Geometry check sheet. Reference: the model listing, model coordinates, mm. A direction names the side the tool comes from. Round coordinates to 2 decimals unless told otherwise and drop trailing zeros. Order: outer loops, then holes, each group sorted by start corner. A loop starts at its lowest first (then second) coordinate and runs counter-clockwise, first axis right, second up. Notation, with made-up numbers: M 32,45.25 L 68,45.25 A15 ccw 68,49.25 Z; hole C 56.25,-14.75 d9. An arc over 180 degrees is marked long. Return JSON: item names as keys, results as strings. Group by question number.
```python
from build123d import *

# Parameters (mm, degrees)
SKETCH1_W           = 70
SKETCH1_H           = 31.9
BOSS_EXTRUDE1_DEPTH = 3
SKETCH2_R           = 1.2
CUT_EXTRUDE1_DEPTH  = 3
SKETCH3_W           = 24
SKETCH3_H           = 22.6
CUT_EXTRUDE2_DEPTH  = 3


with BuildPart() as part:
    # Sketch1 → Boss-Extrude1 (new body)
    with BuildSketch(Plane(origin=(0, 0, 0), x_dir=(1, 0, 0), z_dir=(0, 1, 0))):
        Rectangle(SKETCH1_W, SKETCH1_H)
    extrude(amount=BOSS_EXTRUDE1_DEPTH)

    # Sketch2 → Cut-Extrude1 (cut)
    with BuildSketch(Plane(origin=(0, 3, 0), x_dir=(1, 0, 0), z_dir=(0, 1, 0))):
        with Locations((-29, 13.65)):
            Circle(SKETCH2_R)
    cut_extrude1 = extrude(amount=-CUT_EXTRUDE1_DEPTH, mode=Mode.SUBTRACT)

    # Mirror1: Cut-Extrude1 across plane
    add(cut_extrude1.mirror(Plane.XY), mode=Mode.SUBTRACT)

    # Sketch3 → Cut-Extrude2 (cut)
    with BuildSketch(Plane(origin=(0, 3, 0), x_dir=(1, 0, 0), z_dir=(0, 1, 0))):
        with Locations((-35, 0)):
            Rectangle(SKETCH3_W, SKETCH3_H)
    extrude(amount=-CUT_EXTRUDE2_DEPTH, mode=Mode.SUBTRACT)


solid = part.part
```
Q1. Depth check by flat-ended pin: pin 1 Ø4 at (x, z) = (-1, -0.5) entering from -Y. Enter the tip coordinate at first touch or a pass-through.
Q2. Section check B-B on y = 1.2. Record the cut outline in (x, z), plus the area to 3 significant figures.
Q3. Set-up check for faces 4 (the face through (7, 0, 0)), 5 (the face through (-23, 2, 0)): record each of +Z, -Z, +X, -X, +Y, -Y from which the full face is reachable in a straight line by a thin tool's end or side.
Q4. Release check for a two-part mould opening along Z. For faces 1 (the face through (-28.35, 1.52, 14.66)), 2 (the face through (35, 1, 0)), 3 (the face through (0, 1, 15.95)) record: +Z half, -Z half, draft (parallel to the pull), parting line (faces both ways), or undercut.
Q5. Section check C-C on z = 13.65. Record the cut outline in (x, y), plus the area to 3 significant figures.
Q6. Section check D-D on z = 0. Record the cut outline in (x, y), plus the area to 3 significant figures.
Q7. Section check A-A on x = -29. Record the cut outline in (y, z), plus the area to 3 significant figures.
Q8. Material ranges on line 1 along Z through (x, y) = (-29, 1.45); line 2 along X through (y, z) = (1.55, -13.65); line 3 along X through (y, z) = (2.3, -6), recorded low to high.
Geometry check:
{
 "1": {"pin 1": "stops at y = 0"},
 "2": {"outline": "M -35,-15.95 L 35,-15.95 L 35,15.95 L -35,15.95 L -35,11.3 L -23,11.3 L -23,-11.3 L -35,-11.3 Z; hole C -29,-13.65 d2.4; hole C -29,13.65 d2.4", "area": "1,950 mm^2"},
 "3": {"face 4": "+Z, -Z, +X, -X, -Y", "face 5": "-X, +Y, -Y"},
 "4": {"face 1": "undercut", "face 2": "draft", "face 3": "+Z half"},
 "5": {"outline": "M -35,0 L -30.2,0 L -30.2,3 L -35,3 Z; M -27.8,0 L 35,0 L 35,3 L -27.8,3 Z", "area": "203 mm^2"},
 "6": {"outline": "M -23,0 L 35,0 L 35,3 L -23,3 Z", "area": "174 mm^2"},
 "7": {"outline": "M 0,-15.95 L 3,-15.95 L 3,-14.85 L 0,-14.85 Z; M 0,-12.45 L 3,-12.45 L 3,-11.3 L 0,-11.3 Z; M 0,11.3 L 3,11.3 L 3,12.45 L 0,12.45 Z; M 0,14.85 L 3,14.85 L 3,15.95 L 0,15.95 Z", "area": "13.5 mm^2"},
 "8": {"line 1": "z = -15.95 to -14.85, -12.45 to -11.3, 11.3 to 12.45, 14.85 to 15.95", "line 2": "x = -35 to -30.2, -27.8 to 35", "line 3": "x = -23 to 35"}
}
